Autodesk Inventor part; units mm, degrees
ref_plane "YZ Plane" through (0, 0, 0) normal (1, 0, 0) x (0, 1, 0)
ref_plane "XZ Plane" through (0, 0, 0) normal (0, 1, 0) x (-1, 0, 0)
ref_plane "XY Plane" through (0, 0, 0) normal (0, 0, 1) x (1, 0, 0)
sketch "Sketch1" plane through (0, 0, 0) normal (0, 0, 1) x (1, 0, 0)
  line L0 (0, 0) -> (12.7, 0)
  line L1 (12.7, 0) -> (12.7, 47.625)
  line L2 (12.7, 47.625) -> (0, 47.625)
  line L3 (0, 47.625) -> (0, 0)
  dimension "d0" = 47.625
  dimension "d1" = 12.7
extrude "Extrusion1" add sketch "Sketch1" along normal blind 1.5875
sketch "Sketch2" plane through (0, 0, 1.5875) normal (0, 0, 1) x (1, 0, 0)
  line L0 (12.7, 0) -> (12.7, 47.625)
  line L1 (12.7, 47.625) -> (0, 47.625)
  line L2 (0, 47.625) -> (0, 0)
  point P0 (6.35, 41.275)
  point P1 (6.35, 9.525)
  dimension "d4" = 31.75
  dimension "d6" = 6.35
  dimension "d7" = 6.35
  dimension "d8" = 6.35
hole "Hole1" at (6.35, 41.275, 1.5875) at (6.35, 9.525, 1.5875) direction (0, 0, -1) diameter 5 depth 25.4 tip angle 118
properties part number "SpacerBasket"
Check sheet for the modelled part. Datum: model origin and axes. Units: mm. Round coordinates to 2 decimals unless told otherwise and drop trailing zeros. Loops run counter-clockwise (first coordinate to the right, second up) from the corner with the lowest first, then second, coordinate; pieces in that order, holes last.
1. Sectioned sample at C-C on y = 39.5. Record the boundary of the cut face in (x, z), and give its area (3 significant figures).
2. Sectioned sample at A-A on x = 6.35. Record the boundary of the cut face in (y, z) (1 decimal), and give its area (3 significant figures).
3. Mould release check, pull along X, two halves, no side actions. Record for faces 1 (the flat face through (6, 0, 1)), 2 (the flat face through (0, 24, 1)), 3 (the cylindrical face through (7.87, 11.51, 0.78)): released by +X, released by -X, zero draft, split by the parting line, or undercut.
4. Scan lines: probe 1 along Y at (x, z) = (6.35, 0.45) (3 decimals); probe 2 along Y at (x, z) = (5.5, 0.6) (3 decimals); probe 3 along X at (y, z) = (43, 0.2). Record each from-to range of solid material in increasing order.
5. Sectioned sample at B-B on z = 1.05. Record the boundary of the cut face in (x, y) (3 decimals), and give its area (3 significant figures).
6. Sectioned sample at D-D on y = 9.5. Record the boundary of the cut face in (x, z).
Recorded:
1. outline: (0, 0) - (4.59, 0) - (4.59, 1.59) - (0, 1.59) - close; (8.11, 0) - (12.7, 0) - (12.7, 1.59) - (8.11, 1.59) - close
1. area: 14.6 mm2
2. outline: (0, 0) - (7, 0) - (7, 1.6) - (0, 1.6) - close; (12, 0) - (38.8, 0) - (38.8, 1.6) - (12, 1.6) - close; (43.8, 0) - (47.6, 0) - (47.6, 1.6) - (43.8, 1.6) - close
2. area: 59.7 mm2
3. face 1: zero draft
3. face 2: released by -X
3. face 3: undercut
4. probe 1: y = 0 to 7.025, 12.025 to 38.775, 43.775 to 47.625
4. probe 2: y = 0 to 7.174, 11.876 to 38.924, 43.626 to 47.625
4. probe 3: x = 0 to 4.54, 8.16 to 12.7
5. outline: (0, 0) - (12.7, 0) - (12.7, 47.625) - (0, 47.625) - close; hole circle Ø5 at (6.35, 9.525); hole circle Ø5 at (6.35, 41.275)
5. area: 566 mm2
6. outline: (0, 0) - (3.85, 0) - (3.85, 1.59) - (0, 1.59) - close; (8.85, 0) - (12.7, 0) - (12.7, 1.59) - (8.85, 1.59) - close
